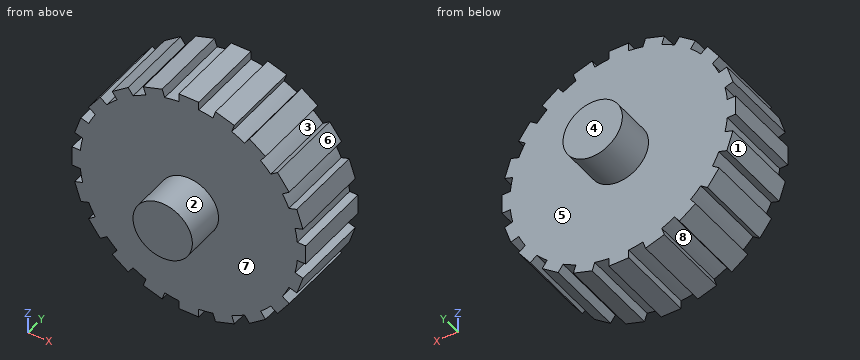
from build123d import *

# Parameters (mm, degrees)
ESQUISSE1_R                  = 7.5
BOSS_EXTRU_1_DEPTH           = 40
ESQUISSE2_R                  = 27.5
BOSS_EXTRU_2_DEPTH           = 20
ESQUISSE3_W                  = 5
ESQUISSE3_H                  = 20
BOSS_EXTRU_3_DEPTH           = 7
R_P_TITION_CIRCULAIRE1_COUNT = 20


with BuildPart() as part:
    # Esquisse1 → Boss.-Extru.1 (new body)
    with BuildSketch(Plane(origin=(0, 0, 0), x_dir=(1, 0, 0), z_dir=(0, 1, 0))):
        with Locations(Location((0, 0, 0), (0, 0, 270))):
            Circle(ESQUISSE1_R)
    extrude(amount=BOSS_EXTRU_1_DEPTH)

    # Esquisse2 → Boss.-Extru.2 (add)
    with BuildSketch(Plane(origin=(0, 10, 0), x_dir=(-1, 0, 0), z_dir=(0, -1, 0))):
        with Locations(Location((0, 0, 0), (0, 0, 90))):
            Circle(ESQUISSE2_R)
    extrude(amount=-BOSS_EXTRU_2_DEPTH)

    # Esquisse3 → Boss.-Extru.3 (add)
    with BuildSketch(Plane.XY.offset(22.5)):
        with Locations((0, 20)):
            Rectangle(ESQUISSE3_W, ESQUISSE3_H)
    boss_extru_3 = extrude(amount=BOSS_EXTRU_3_DEPTH)

    # Répétition circulaire1: Boss.-Extru.3 ×20 about axis
    r_p_tition_circulaire1_axis = Axis((0, 0, 0), (0, 1, 0))
    for i in range(1, R_P_TITION_CIRCULAIRE1_COUNT):
        add(boss_extru_3.rotate(r_p_tition_circulaire1_axis, i * 360 / R_P_TITION_CIRCULAIRE1_COUNT))


solid = part.part
The listing builds one solid part. Answer for the finished solid, in the listing's coordinates (mm). Face numbers are marked on the shaded views. A direction names the side the tool comes from. Coordinates: 2 decimals unless noted, no trailing zeros. Loops run counter-clockwise (first coordinate to the right, second up) from the corner with the lowest first, then second, coordinate; pieces in that order, holes last. Notation, with made-up numbers: (67, 55.5) -> (84, 55.5) arc R17 ccw to (84, 71.5) -> close; hole circle Ø7 at (-13.75, -22.5). An arc over 180 degrees is marked (long way). Answer in a Markdown table with one row per item. Add a question column.
1. Determine the mould class of the marked faces 1, 2 and 3 for opening direction Z: +Z half, -Z half, draft (parallel to the pull), parting line (faces both ways), or undercut.
2. The part is cut by section D-D, the plane z = -17. Write down the section's boundary in (x, y), then the cut area to 3 significant figures.
3. The part is cut by section A-A, the plane z = 0. Write down the section's boundary in (x, y), then the cut area to 3 significant figures.
4. Consider line 1 (Z direction, x = -24, y = 13); line 2 (Y direction, x = 9, z = 0); line 3 (Z direction, x = 6, y = 25.5). Determine where each line is inside the solid, lowest interval first. Write a range as [from, to].
5. The part is cut by section B-B, the plane x = 0. Write down the section's boundary in (y, z), then the cut area to 3 significant figures.
6. For the marked faces 4, 5, 6, 7 and 8, determine the directions among +Z, -Z, +X, -X, +Y, -Y from which every point of the face is accessible in a straight line to the end or side of a thin tool.
7. Flat-ended cylindrical pins translate along their axes: P1, Ø2.5, axis at x = 28, y = 15, coming from the +Z side; P2, Ø2.5, axis at x = 28, y = 24, coming from the -Z side; P3, Ø10, axis at x = -2, z = -8.5, coming from the +Y side; P4, Ø8, axis at x = -8, y = 26, coming from the -Z side. Find the tip coordinate at first contact, or state that the pin passes through.
8. The part is cut by section C-C, the plane y = 35. Write down the section's boundary in (x, z).
Answer below:
| question | item | result |
|---|---|---|
| 1 | face 1 | -Z half |
| 1 | face 2 | parting line |
| 1 | face 3 | undercut |
| 2 | outline | (-24.11, 10) -> (24.11, 10) -> (24.11, 30) -> (-24.11, 30) -> close |
| 2 | area | 965 mm2 |
| 3 | outline | (-29.5, 10) -> (-7.5, 10) -> (-7.5, 0) -> (7.5, 0) -> (7.5, 10) -> (29.5, 10) -> (29.5, 30) -> (7.5, 30) -> (7.5, 40) -> (-7.5, 40) -> (-7.5, 30) -> (-29.5, 30) -> close |
| 3 | area | 1,480 mm2 |
| 4 | line 1 | [-17.16, -14.35], [-13.43, 13.43], [14.35, 17.16] |
| 4 | line 2 | [10, 30] |
| 4 | line 3 | [-26.84, 26.84] |
| 5 | outline | (0, -7.5) -> (10, -7.5) -> (10, -29.5) -> (30, -29.5) -> (30, -7.5) -> (40, -7.5) -> (40, 7.5) -> (30, 7.5) -> (30, 29.5) -> (10, 29.5) -> (10, 7.5) -> (0, 7.5) -> close |
| 5 | area | 1,480 mm2 |
| 6 | face 4 | +Z, -Z, +X, -X, +Y |
| 6 | face 5 | +Y |
| 6 | face 6 | +Z, +X, +Y, -Y |
| 6 | face 7 | -Y |
| 6 | face 8 | +Y, -Y |
| 7 | P1 | z = 11.49 |
| 7 | P2 | z = -11.49 |
| 7 | P3 | y = 40 |
| 7 | P4 | z = -28.83 |
| 8 | outline | circle Ø15 at (0, 0) |
